Could you check a few things on this model? Use its own coordinates, in mm. Face numbers are marked on the shaded views. A direction names the side the tool comes from. Coordinates: 2 decimals unless noted, no trailing zeros. Loops run counter-clockwise (first coordinate to the right, second up) from the corner with the lowest first, then second, coordinate; pieces in that order, holes last. Notation, with made-up numbers: (-40, -32) - (-6, -32) arc R12 ccw to (-6, -16) - close; hole circle Ø5 at (-17, -8.5). An arc over 180 degrees is marked (long way). One line per question, with ' | ' between items. Start each with the question number.
1. Please list where these lines run through material, in increasing order: L1, parallel to X at y = 0, z = 2.5; L2, parallel to Z at x = -21.25, y = -11.15; L3, parallel to Y at x = -25, z = -1.5. Write a range as [from, to].
2. I want a section at B-B, the plane x = 21.25. Write out the boundary of the cut face in (y, z).
3. We'd pull the mould along X, two halves only. Please class the marked faces 4, 5, 6 and 7: pulls with the +X half, pulls with the -X half, needs draft (parallel to the pull), parting line crosses it, or undercut.
4. Which directions (+Z, -Z, +X, -X, +Y, -Y) give clear straight access to the entire face, cutting with the end or side of a thin tool? Please do the marked faces 1, 2 and 3.
5. I want a section at D-D, the plane x = -16.5. Write out the boundary of the cut face in (y, z).
6. I want a section at A-A, the plane z = 0. Count the separate pieces of the cut face and the enclosed holes in it, then the cut area to 3 significant figures.
7. I'm going to push flat-ended pins straight in: P1, Ø1.5, axis at x = -17.5, y = -13, coming from the +Z side; P2, Ø3.5, axis at x = -20, z = 2, coming from the +Y side; P3, Ø5, axis at x = -9.5, z = -4.5, coming from the +Y side; P4, Ø6.5, axis at y = -9.5, z = 0.5, coming from the +X side. Where does each tip first touch, or does it pass through?
from build123d import *

# Parameters (mm, degrees)
SKETCH1_R           = 10
BOSS_EXTRUDE1_DEPTH = 4
SKETCH2_R           = 9.25
CUT_EXTRUDE2_DEPTH  = 0.5
SKETCH6_R           = 14.1
SKETCH6_R_2         = 10
BOSS_EXTRUDE4_DEPTH = 6.5
SKETCH7_OUTSIDE_W   = 27.678
SKETCH7_OUTSIDE_H   = 43.378
CUT_EXTRUDE6_DEPTH  = 28.5
SKETCH8_R           = 4
CUT_EXTRUDE7_DEPTH  = 7
SKETCH11_W          = 25
SKETCH11_H          = 1.75
CUT_EXTRUDE8_DEPTH  = 29.2
CUT_EXTRUDE9_DEPTH  = 3.5
SKETCH9_R           = 5.5
SKETCH9_R_2         = 4
BOSS_EXTRUDE5_DEPTH = 4.3
SKETCH10_R          = 5.5
SKETCH10_R_2        = 4
BOSS_EXTRUDE6_DEPTH = 1
SKETCH13_W          = 11
SKETCH13_H          = 9
CUT_EXTRUDE10_DEPTH = 3
SKETCH14_R          = 2.5
CUT_EXTRUDE11_DEPTH = 2
CHAMFER1_SIZE       = 2
FILLET1_R           = 1


with BuildPart() as part:
    # Sketch1 → Boss-Extrude1 (new body, symmetric)
    with BuildSketch(Plane.XY):
        Circle(SKETCH1_R)
    extrude(amount=BOSS_EXTRUDE1_DEPTH, both=True)

    # Sketch2 → Cut-Extrude2 (cut)
    with BuildSketch(Plane.XY.offset(4)):
        Circle(SKETCH2_R)
    cut_extrude2 = extrude(amount=-CUT_EXTRUDE2_DEPTH, mode=Mode.SUBTRACT)

    # Mirror1: Cut-Extrude2 across plane
    add(cut_extrude2.mirror(Plane.XY), mode=Mode.SUBTRACT)

    # Sketch6 → Boss-Extrude4 (add, symmetric)
    with BuildSketch(Plane.XY):
        Circle(SKETCH6_R)
        Circle(SKETCH6_R_2, mode=Mode.SUBTRACT)
        with BuildLine():
            ThreePointArc((4.2e-08, -14.1), (-9.9702056, -9.97020563), (-14.1, 0))
            Line((-14.1, 0), (-15, -9.6))
            Line((-15, -9.6), (-27.5, -9.6))
            Line((-27.5, -9.6), (-27.5, -14.6))
            Line((-27.5, -14.6), (-12.5, -14.6))
            Line((-12.5, -14.6), (-12.5, -14.1))
            Line((-12.5, -14.1), (4.2e-08, -14.1))
        make_face()
        with BuildLine():
            Line((15, -9.6), (14.1, 0))
            ThreePointArc((14.1, 0), (9.97020563, -9.9702056), (4.2e-08, -14.1))
            Line((4.2e-08, -14.1), (12.5, -14.1))
            Line((12.5, -14.1), (12.5, -14.6))
            Line((12.5, -14.6), (27.5, -14.6))
            Line((27.5, -14.6), (27.5, -9.6))
            Line((27.5, -9.6), (15, -9.6))
        make_face()
    extrude(amount=BOSS_EXTRUDE4_DEPTH, both=True)

    # Sketch7 outside → Cut-Extrude6 (cut, symmetric)
    with BuildSketch(Plane(origin=(0, 0, 0), x_dir=(0, 0, -1), z_dir=(1, 0, 0))):
        with Locations((0, -0.25)):
            Rectangle(SKETCH7_OUTSIDE_W, SKETCH7_OUTSIDE_H)
        Polygon((-6.5, -9.6), (-4.75, 0), (-4.75, 14.1), (4.75, 14.1), (4.75, 0), (6.5, -9.6), (6.5, -14.6), (-6.5, -14.6), align=None, mode=Mode.SUBTRACT)
    extrude(amount=CUT_EXTRUDE6_DEPTH, both=True, mode=Mode.SUBTRACT)

    # Sketch8 → Cut-Extrude7 (cut)
    with BuildSketch(Plane.XY.offset(3.5)):
        Circle(SKETCH8_R)
    extrude(amount=-CUT_EXTRUDE7_DEPTH, mode=Mode.SUBTRACT)

    # Sketch11 → Cut-Extrude8 (cut, through all)
    with BuildSketch(Plane.XZ.offset(14.1)):
        with Locations((0, 5.625)):
            Rectangle(SKETCH11_W, SKETCH11_H)
        with Locations((0, -5.625)):
            Rectangle(SKETCH11_W, SKETCH11_H)
    extrude(amount=-CUT_EXTRUDE8_DEPTH, mode=Mode.SUBTRACT)

    # Sketch12 → Cut-Extrude9 (cut)
    with BuildSketch(Plane.XY.offset(4.75)):
        with BuildLine():
            ThreePointArc((0, -14.1), (-7.308364514, -12.058101349), (-12.5, -6.523802572))
            Line((-12.5, -6.523802572), (-12.5, -14.1))
            Line((-12.5, -14.1), (0, -14.1))
        make_face()
        with BuildLine():
            ThreePointArc((12.5, -6.523802572), (7.308364514, -12.058101349), (0, -14.1))
            Line((0, -14.1), (12.5, -14.1))
            Line((12.5, -14.1), (12.5, -6.523802572))
        make_face()
    cut_extrude9 = extrude(amount=-CUT_EXTRUDE9_DEPTH, mode=Mode.SUBTRACT)

    # Mirror2: Cut-Extrude9 across plane
    add(cut_extrude9.mirror(Plane.XY), mode=Mode.SUBTRACT)

    # Sketch9 → Boss-Extrude5 (add)
    with BuildSketch(Plane.XY.offset(3.5)):
        Circle(SKETCH9_R)
        Circle(SKETCH9_R_2, mode=Mode.SUBTRACT)
    extrude(amount=BOSS_EXTRUDE5_DEPTH)

    # Sketch10 → Boss-Extrude6 (add)
    with BuildSketch(Plane(origin=(0, 0, -3.5), x_dir=(-1, 0, 0), z_dir=(0, 0, -1))):
        Circle(SKETCH10_R)
        Circle(SKETCH10_R_2, mode=Mode.SUBTRACT)
    extrude(amount=BOSS_EXTRUDE6_DEPTH)

    # Sketch13 → Cut-Extrude10 (cut)
    with BuildSketch(Plane.XZ.offset(14.6)):
        with Locations((-20, 0)):
            Rectangle(SKETCH13_W, SKETCH13_H)
        with Locations((20, 0)):
            Rectangle(SKETCH13_W, SKETCH13_H)
    extrude(amount=-CUT_EXTRUDE10_DEPTH, mode=Mode.SUBTRACT)

    # Sketch14 → Cut-Extrude11 (cut)
    with BuildSketch(Plane.XZ.offset(11.6)):
        with Locations((21.25, 0)):
            Circle(SKETCH14_R)
        with Locations((-21.25, 0)):
            Circle(SKETCH14_R)
    extrude(amount=-CUT_EXTRUDE11_DEPTH, mode=Mode.SUBTRACT)

    # Chamfer1
    chamfer1_edges = [part.edges().sort_by_distance(p)[0] for p in [
        (-27.5, -12.1, -6.5),
        (27.5, -12.1, 6.5),
        (-27.5, -12.1, 6.5),
        (27.5, -12.1, -6.5),
    ]]
    chamfer(chamfer1_edges, length=CHAMFER1_SIZE)

    # Fillet1
    fillet1_edges = [part.edges().sort_by_distance(p)[0] for p in [
        (-15, -9.6, 0),
        (-12.5, -6.523802572, 3),
        (15, -9.6, 0),
        (12.5, -6.523802572, 3),
        (-12.5, -6.523802572, -3),
        (12.5, -6.523802572, -3),
    ]]
    fillet(fillet1_edges, radius=FILLET1_R)


solid = part.part
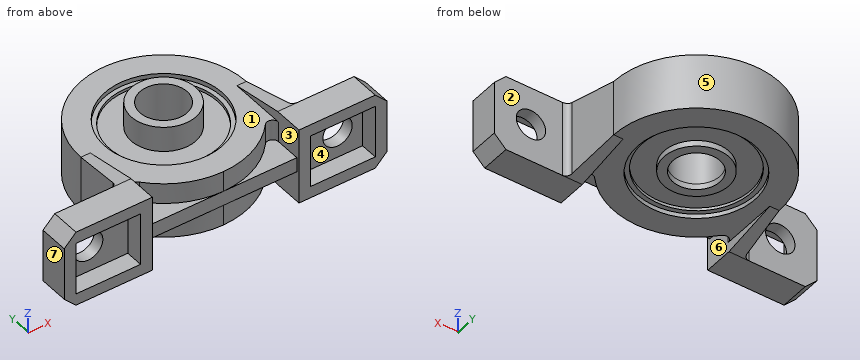
Results are:
1) L1: x = [-14.1, -4], [4, 14.1] | L2: z = [-6.5, -2.5], [2.5, 6.5] | L3: y = [-11.6, -9.6]
2) outline: (-14.6, -6.5) - (-9.6, -6.5) - (-9.6, -2.5) - (-11.6, -2.5) - (-11.6, -4.5) - (-14.6, -4.5) - close; (-14.6, 4.5) - (-11.6, 4.5) - (-11.6, 2.5) - (-9.6, 2.5) - (-9.6, 6.5) - (-14.6, 6.5) - close
3) face 4: undercut | face 5: parting line crosses it | face 6: undercut | face 7: pulls with the -X half
4) face 1: +Z | face 2: +Z, -Z, +X, +Y | face 3: -Y
5) outline: (-14.6, -6.5) - (-9.6, -6.5) - (-9.6, 6.5) - (-14.6, 6.5) - (-14.6, 4.5) - (-11.6, 4.5) - (-11.6, -4.5) - (-14.6, -4.5) - close
6) separate pieces: 3 | enclosed holes: 1 | area: 718 mm2
7) P1: stops at z = 6.5 | P2: stops at y = -9.6 | P3: stops at y = 12.24 | P4: stops at x = 27.5
